from build123d import *

# Parameters (mm, degrees)
F1_DEPTH = 25.4
F3_DEPTH = 25.4
F4_W     = 10.353053
F4_H     = 12.504167
F5_DEPTH = 25.4


with BuildPart() as f1:
    # F0 (on Front) → F1 (new body)
    with BuildSketch(Plane.XZ):
        Polygon((18.569692, 7.642571), (-25.87954, 7.38124), (-26.865089, -24.35346), (17.533206, -25.732289), align=None)
    extrude(amount=F1_DEPTH)

    # F2 (on face) → F3 (cut)
    with BuildSketch(Plane.XZ.offset(25.4)):
        Polygon((18.569692, 7.642571), (-2.184069, 7.520553), (17.533206, -25.732289), align=None)
    extrude(amount=-F3_DEPTH, mode=Mode.SUBTRACT)

    # F4 (on face) → F5 (join)
    with BuildSketch(Plane(origin=(1.683383, 0, 0.998162), x_dir=(0, 1, 0), z_dir=(0.860157, 0, 0.51003))):
        with Locations((-5.176526, -24.824175)):
            Rectangle(F4_W, F4_H)
    extrude(amount=F5_DEPTH)


solid = f1.part
Verification items for the finished model (mm, model axes). A direction names the side the tool comes from. Give positions to 0.01 mm unless a question says otherwise; leave off trailing zeros. Loops run counter-clockwise (first coordinate to the right, second up) from the corner with the lowest first, then second, coordinate; pieces in that order, holes last.
1. Cross-section at D-D on x = 29. Record the cut outline in (y, z), and give its area (3 significant figures).
Derived:
outline: (-10.35, -18.93) - (0, -18.93) - (0, -4.4) - (-10.35, -4.4) - close
area: 151 mm2
2. Cross-section at A-A on z = -11. Record the cut outline in (x, y), and give its area (3 significant figures).
Derived:
outline: (-26.45, -25.4) - (8.8, -25.4) - (8.8, 0) - (-26.45, 0) - close; (17.86, -10.35) - (38.33, -10.35) - (38.33, 0) - (17.86, 0) - close
area: 1,110 mm2
3. Release check for a two-part mould opening along X. For faces 1 (the flat face through (-10, 0, -9)), 2 (the flat face through (21.93, -5.25, -8.59)), 3 (the flat face through (36.148, -5.249, -7.324)) record: +X half, -X half, draft (parallel to the pull), parting line (faces both ways), or undercut.
Derived:
face 1: draft
face 2: undercut
face 3: +X half
4. Material ranges on probe 1 along Y at (x, z) = (20, -14.5); probe 2 along X at (y, z) = (-10.25, -8); probe 3 along Z at (x, y) = (8, -11.75), recorded low to high.
Derived:
probe 1: y = -10.35 to 0
probe 2: x = -26.36 to 7.02, 22.92 to 36.55
probe 3: z = -25.44 to -9.65
5. Tool access check on faces 4 (the flat face through (25, -10.353, -14)), 5 (the flat face through (5.346, -12.878, -5.178)), 6 (the flat face through (28.3, -5.25, -19.35)). Record the directions out of +Z, -Z, +X, -X, +Y, -Y that give a thin tool (end or side, any length) a straight path to the whole face; none if there is none.
Derived:
face 4: +Z, +X, -Y
face 5: +Z, -Y
face 6: -Z, +X, +Y, -Y
6. Cross-section at C-C on z = -18. Record the cut outline in (x, y).
Derived:
outline: (-26.67, -25.4) - (12.95, -25.4) - (12.95, -10.35) - (30.57, -10.35) - (30.57, 0) - (-26.67, 0) - close
7. Go/stop test with flat-tipped pins: P1, Ø3, axis at x = 25, y = -9.5, coming from the +Z side; P2, Ø6, axis at x = 27.5, y = -8.5, coming from the +Z side; P3, Ø1.5, axis at x = 21, y = -7.5, coming from the -Z side; P4, Ø8, axis at x = -13, z = -2, coming from the +Y side. Record where each tip stops, or that it passes through.
Derived:
P1: stops at z = -5.88
P2: stops at z = -3.51
P3: stops at z = -24.12
P4: stops at y = 0
